from build123d import *

# Parameters (mm, degrees)
F0_R     = 3.95
F1_DEPTH = 12
F2_R     = 1.55
F3_DEPTH = 12.001
F4_R     = 0.5


with BuildPart() as f1:
    # F0 (on Top) → F1 (new body)
    with BuildSketch(Plane.XY):
        Circle(F0_R)
    extrude(amount=F1_DEPTH)

    # F2 (on face) → F3 (cut, through all)
    with BuildSketch(Plane(origin=(0, 0, 0), x_dir=(1, 0, 0), z_dir=(0, 0, -1))):
        Circle(F2_R)
    extrude(amount=-F3_DEPTH, mode=Mode.SUBTRACT)

    # F4
    f4_edges = [f1.edges().sort_by_distance(p)[0] for p in [
        (-3.95, 0, 0),
        (-3.95, 0, 12),
    ]]
    fillet(f4_edges, radius=F4_R)


solid = f1.part
Check sheet for the modelled part. Datum: model origin and axes. Units: mm. Give positions to 0.01 mm unless a question says otherwise; leave off trailing zeros. Write each loop counter-clockwise with the first axis right and the second up, starting at its lowest first coordinate (ties: lowest second). Pieces come first, ordered by that corner, then holes. Notation, with made-up numbers: M -36.75,58.5 L -15.75,58.5 A25 ccw -15.75,95.5 Z; hole C 0.5,45.5 d10. An arc over 180 degrees is marked long. Use one line per item in the form item = value.
(1) Section check A-A on y = 0. Record the boundary of the cut face in (x, z).
Answer block:
outline = M -3.95,0.5 A0.5 ccw -3.45,0 L -1.55,0 L -1.55,12 L -3.45,12 A0.5 ccw -3.95,11.5 Z; M 1.55,0 L 3.45,0 A0.5 ccw 3.95,0.5 L 3.95,11.5 A0.5 ccw 3.45,12 L 1.55,12 Z
(2) Section check C-C on z = 11.25. Record the boundary of the cut face in (x, y), plus the area to 3 significant figures.
Answer block:
outline = C 0,0 d7.9; hole C 0,0 d3.1
area = 41.5 mm2
(3) Material ranges on line 1 along Y through (x, z) = (0, 3); line 2 along Y through (x, z) = (0.75, 5.5); line 3 along X through (y, z) = (-1.25, 1), recorded low to high.
Answer block:
line_1 = -3.95 to -1.55, 1.55 to 3.95
line_2 = -3.88 to -1.36, 1.36 to 3.88
line_3 = -3.75 to -0.92, 0.92 to 3.75
(4) Draft check along Y on faces 1 (the cylindrical face through (-3.135, -2.404, 5.923)), 2 (the flat face through (0, 2, 12)), 3 (the cylindrical face through (0.715, 1.375, 5.916)). Enter one of: pulls with the +Y half, pulls with the -Y half, needs draft (parallel to the pull), parting line crosses it, or undercut.
Answer block:
face_1 = parting line crosses it
face_2 = needs draft
face_3 = undercut
